Verification items for the finished model (mm, model axes). Round coordinates to 2 decimals unless told otherwise and drop trailing zeros. Loops run counter-clockwise (first coordinate to the right, second up) from the corner with the lowest first, then second, coordinate; pieces in that order, holes last. Notation, with made-up numbers: (6.5, -35) -> (57.5, -35) arc R29 cw to (57.5, 4) -> close; hole circle Ø9 at (52, -18.5). An arc over 180 degrees is marked (long way). Use CSV: the item, a comma, the result in double quotes. Start each with the question number.
```python
from build123d import *

# Parameters (mm, degrees)
SKETCH1_R           = 3.175
BOSS_EXTRUDE1_DEPTH = 3.81
SKETCH2_R           = 3.175
BOSS_EXTRUDE2_DEPTH = 2.54
FILLET1_R           = 50.8
SKETCH3_W           = 15.24
SKETCH3_H           = 25.4
CUT_EXTRUDE1_DEPTH  = 7.35


with BuildPart() as part:
    # Sketch1 → Boss-Extrude1 (new body)
    with BuildSketch(Plane(origin=(0, 0, 0), x_dir=(1, 0, 0), z_dir=(0, 1, 0))):
        Polygon((-76.2, -50.8), (-38.1, -88.9), (38.1, -88.9), (76.2, -50.8), (76.2, 88.9), (-76.2, 88.9), align=None)
        with Locations((0, 76.2)):
            Circle(SKETCH1_R, mode=Mode.SUBTRACT)
        with Locations((0, -76.2)):
            Circle(SKETCH1_R, mode=Mode.SUBTRACT)
    extrude(amount=BOSS_EXTRUDE1_DEPTH)

    # Sketch2 → Boss-Extrude2 (add)
    with BuildSketch(Plane.XZ):
        Polygon((-69.85, 48.169743879), (-69.85, -82.55), (69.85, -82.55), (69.85, 48.169743879), (35.469743879, 82.55), (-35.469743879, 82.55), align=None)
        with Locations((0, 76.2)):
            Circle(SKETCH2_R, mode=Mode.SUBTRACT)
        with Locations((0, -76.2)):
            Circle(SKETCH2_R, mode=Mode.SUBTRACT)
    extrude(amount=BOSS_EXTRUDE2_DEPTH)

    # Fillet1
    fillet1_edges = [part.edges().sort_by_distance(p)[0] for p in [
        (76.2, 1.905, 50.8),
        (38.1, 1.905, 88.9),
        (-38.1, 1.905, 88.9),
        (-76.2, 1.905, 50.8),
    ]]
    fillet(fillet1_edges, radius=FILLET1_R)

    # Sketch3 → Cut-Extrude1 (cut, through all)
    with BuildSketch(Plane(origin=(0, 3.81, 0), x_dir=(1, 0, 0), z_dir=(0, 1, 0))):
        with Locations((-12.7, 25.4)):
            Rectangle(SKETCH3_W, SKETCH3_H)
    extrude(amount=-CUT_EXTRUDE1_DEPTH, mode=Mode.SUBTRACT)


solid = part.part
```
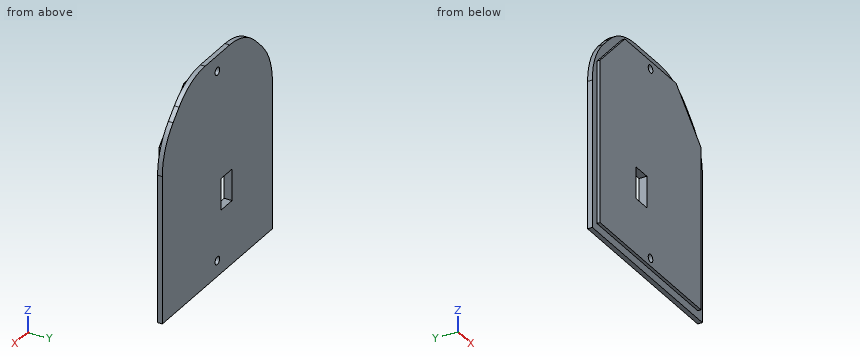
Q1. Cross-section at B-B (y = 1.75). Record the boundary of the cut face in (x, z) (3 decimals), and give its area (3 significant figures).
Q2. Cross-section at C-C (z = -76.2). Record the boundary of the cut face in (x, y) (3 decimals), and give its area (3 significant figures).
Q3. Depth check by flat-ended pin: pin 1 Ø1.5 at (y, z) = (-1, 4) entering from +X; pin 2 Ø1.3 at (x, y) = (33, -1.5) entering from -Z. Enter the tip coordinate at first touch or a pass-through.
Q4. Thickness scan on L1, parallel to Z at x = 0, y = 1 (3 decimals); L2, parallel to Z at x = 0, y = -0.5 (3 decimals); L3, parallel to Z at x = -19, y = 3.5. Record the ranges inside material, lowest first. Write a range as from..to.
Q5. Cross-section at A-A (x = 0). Record the boundary of the cut face in (y, z) (3 decimals).
Q6. Cross-section at D-D (z = 15.5). Record the boundary of the cut face in (x, y).
Answer list:
1,outline,"(-76.2, -88.9) -> (76.2, -88.9) -> (76.2, 29.758) arc R50.8 ccw to (61.321, 65.679) -> (52.979, 74.021) arc R50.8 ccw to (17.058, 88.9) -> (-17.058, 88.9) arc R50.8 ccw to (-52.979, 74.021) -> (-61.321, 65.679) arc R50.8 ccw to (-76.2, 29.758) -> close; hole (-20.32, -38.1) -> (-5.08, -38.1) -> (-5.08, -12.7) -> (-20.32, -12.7) -> close; hole circle Ø6.35 at (0, -76.2); hole circle Ø6.35 at (0, 76.2)"
1,area,"25,000 mm2"
2,outline,"(-76.2, 0) -> (-69.85, 0) -> (-69.85, -2.54) -> (-3.175, -2.54) -> (-3.175, 3.81) -> (-76.2, 3.81) -> close; (3.175, -2.54) -> (69.85, -2.54) -> (69.85, 0) -> (76.2, 0) -> (76.2, 3.81) -> (3.175, 3.81) -> close"
2,area,"895 mm2"
3,pin 1,"stops at x = 69.85"
3,pin 2,"stops at z = -82.55"
4,L1,"z = -88.9..-79.375, -73.025..73.025, 79.375..88.9"
4,L2,"z = -82.55..-79.375, -73.025..73.025, 79.375..82.55"
4,L3,"z = -88.9..-38.1, -12.7..88.86"
5,outline,"(-2.54, -82.55) -> (0, -82.55) -> (0, -88.9) -> (3.81, -88.9) -> (3.81, -79.375) -> (-2.54, -79.375) -> close; (-2.54, -73.025) -> (3.81, -73.025) -> (3.81, 73.025) -> (-2.54, 73.025) -> close; (-2.54, 79.375) -> (3.81, 79.375) -> (3.81, 88.9) -> (0, 88.9) -> (0, 82.55) -> (-2.54, 82.55) -> close"
6,outline,"(-76.2, 0) -> (-69.85, 0) -> (-69.85, -2.54) -> (69.85, -2.54) -> (69.85, 0) -> (76.2, 0) -> (76.2, 3.81) -> (-76.2, 3.81) -> close"
